Geometry: final body of the model. Coordinates: model frame, mm. Coordinates: 2 decimals unless noted, no trailing zeros. Write each loop counter-clockwise with the first axis right and the second up, starting at its lowest first coordinate (ties: lowest second). Pieces come first, ordered by that corner, then holes. Notation, with made-up numbers: (31, -30) - (60, -30) arc R37 ccw to (60, 6) - close; hole circle Ø7 at (-9, 66). An arc over 180 degrees is marked (long way). Put each result on its own line as item: value.
```python
from build123d import *

# Parameters (mm, degrees)
SKETCH1_R           = 24
SKETCH1_R_2         = 11.5
BOSS_EXTRUDE1_DEPTH = 2
SKETCH2_R           = 1.7
CUT_EXTRUDE1_DEPTH  = 3
CHAMFER2_SIZE       = 0.3


with BuildPart() as part:
    # Sketch1 → Boss-Extrude1 (new body)
    with BuildSketch(Plane(origin=(0, 0, 0), x_dir=(1, 0, 0), z_dir=(0, 1, 0))):
        Circle(SKETCH1_R)
        Circle(SKETCH1_R_2, mode=Mode.SUBTRACT)
    extrude(amount=BOSS_EXTRUDE1_DEPTH)

    # Sketch2 → Cut-Extrude1 (cut, through all)
    with BuildSketch(Plane(origin=(0, 2, 0), x_dir=(1, 0, 0), z_dir=(0, 1, 0))):
        with Locations((-20, 0)):
            Circle(SKETCH2_R)
        with Locations((-10, 17.320508076)):
            Circle(SKETCH2_R)
        with Locations((10, 17.320508076)):
            Circle(SKETCH2_R)
        with Locations((20, 0)):
            Circle(SKETCH2_R)
        with Locations((10, -17.320508076)):
            Circle(SKETCH2_R)
        with Locations((-10, -17.320508076)):
            Circle(SKETCH2_R)
    extrude(amount=-CUT_EXTRUDE1_DEPTH, mode=Mode.SUBTRACT)

    # Chamfer2
    chamfer2_edges = [part.edges().sort_by_distance(p)[0] for p in [
        (-21.7, 0, 0),
        (-21.7, 2, 0),
        (-24, 0, 0),
        (-11.7, 0, 17.320508076),
        (-11.7, 2, 17.320508076),
        (8.3, 0, 17.320508076),
        (8.3, 2, 17.320508076),
        (18.3, 0, 0),
        (18.3, 2, 0),
        (8.3, 0, -17.320508076),
        (8.3, 2, -17.320508076),
        (-11.7, 0, -17.320508076),
        (-11.7, 2, -17.320508076),
        (-24, 2, 0),
        (-11.5, 0, 0),
        (-11.5, 2, 0),
    ]]
    chamfer(chamfer2_edges, length=CHAMFER2_SIZE)


solid = part.part
```
1. Mould query, pull axis X, two halves, no side actions, for faces 1 (the flat face through (-11, 0, 5)), 2 (the cylindrical face through (-9.22, 1.01, 18.83)), 3 (the cylindrical face through (-23.977, 0.99, -1.055)). Classes: +X half, -X half, draft (parallel to the pull), parting line (faces both ways), or undercut.
Answer below:
face 1: draft
face 2: undercut
face 3: parting line
2. Section query C-C (x = -10). Count the separate pieces of the cut face and the enclosed holes in it, then the cut area to 3 significant figures.
Answer below:
separate pieces: 4
enclosed holes: 0
area: 50.0 mm²
3. Pin query (flat end, axial travel): pin 1 Ø3 at (x, z) = (-20, 0) entering from -Y. Return the tip coordinate at first contact, or that it passes through.
Answer below:
pin 1: passes through
4. Section query B-B (y = 1.15). Return loops of the section in (x, z).
Answer below:
outline: circle Ø48 at (0, 0); hole circle Ø3.4 at (-20, 0); hole circle Ø3.4 at (-10, -17.32); hole circle Ø3.4 at (-10, 17.32); hole circle Ø23 at (0, 0); hole circle Ø3.4 at (10, -17.32); hole circle Ø3.4 at (10, 17.32); hole circle Ø3.4 at (20, 0)
5. Section query A-A (x = 0). Return loops of the section in (y, z), then the cut area to 3 significant figures.
Answer below:
outline: (0, -23.7) - (0.3, -24) - (1.7, -24) - (2, -23.7) - (2, -11.8) - (1.7, -11.5) - (0.3, -11.5) - (0, -11.8) - close; (0, 11.8) - (0.3, 11.5) - (1.7, 11.5) - (2, 11.8) - (2, 23.7) - (1.7, 24) - (0.3, 24) - (0, 23.7) - close
area: 49.6 mm²
6. Ray query, probe 1 along Z at (x, y) = (-10, 0.6); probe 2 along X at (y, z) = (1.55, 16.5); probe 3 along X at (y, z) = (0.8, 17.5). Return the intervals inside material, ascending. Write a range as from..to.
Answer below:
probe 1: z = -21.82..-19.02, -15.62..-5.68, 5.68..15.62, 19.02..21.82
probe 2: x = -17.43..-11.49, -8.51..8.51, 11.49..17.43
probe 3: x = -16.42..-11.69, -8.31..8.31, 11.69..16.42
